Geometry: final body of the model. Coordinates: model frame, mm. Face numbers are marked on the shaded views. A direction names the side the tool comes from. Coordinates: 2 decimals unless noted, no trailing zeros. Loops run counter-clockwise (first coordinate to the right, second up) from the corner with the lowest first, then second, coordinate; pieces in that order, holes last. Notation, with made-up numbers: (28.25, 89) - (68.25, 89) arc R27 ccw to (68.25, 126) - close; hole circle Ø8 at (7, -12.75). An arc over 180 degrees is marked (long way). Answer in a Markdown table with one row per item.
from build123d import *

# Parameters (mm, degrees)
F1_DEPTH = 10.16
F3_DEPTH = 381
F5_DEPTH = 7.62


with BuildPart() as f1:
    # F0 (on Top) → F1 (new body)
    with BuildSketch(Plane.XY):
        with BuildLine():
            Line((-76.2, -76.2), (76.2, -76.2))
            ThreePointArc((76.2, -76.2), (94.1605122421, -68.7605122421), (101.6, -50.8))
            Line((101.6, -50.8), (101.6, 50.8))
            ThreePointArc((101.6, 50.8), (94.1605122421, 68.7605122421), (76.2, 76.2))
            Line((76.2, 76.2), (-76.2, 76.2))
            ThreePointArc((-76.2, 76.2), (-94.1605122421, 68.7605122421), (-101.6, 50.8))
            Line((-101.6, 50.8), (-101.6, -50.8))
            ThreePointArc((-101.6, -50.8), (-94.1605122421, -68.7605122421), (-76.2, -76.2))
        make_face()
    extrude(amount=-F1_DEPTH)

    # F2 (on face) → F3 (join)
    with BuildSketch(Plane.XY):
        with BuildLine():
            Line((-14.3209369853, 21.4582365006), (14.3209369853, 21.4582365006))
            Line((14.3209369853, 21.4582365006), (14.3209369853, 21.8244272492))
            ThreePointArc((14.3209369853, 21.8244272492), (6.4622604496, 29.6831037849), (14.3209369853, 37.5417803207))
            Line((14.3209369853, 37.5417803207), (14.3209369853, 37.9079710692))
            Line((14.3209369853, 37.9079710692), (-14.3209369853, 37.9079710692))
            Line((-14.3209369853, 37.9079710692), (-14.3209369853, 37.7833950656))
            ThreePointArc((-14.3209369853, 37.7833950656), (-8.5931660912, 35.410874679), (-6.2206457047, 29.6831037849))
            ThreePointArc((-6.2206457047, 29.6831037849), (-8.5931660912, 23.9553328908), (-14.3209369853, 21.5828125043))
            Line((-14.3209369853, 21.5828125043), (-14.3209369853, 21.4582365006))
        make_face()
        with BuildLine():
            ThreePointArc((14.3209369853, 37.5417803207), (6.4622604496, 29.6831037849), (14.3209369853, 21.8244272492))
            Line((14.3209369853, 21.8244272492), (14.3209369853, 37.5417803207))
        make_face()
        with BuildLine():
            Line((14.3209369853, 37.5417803207), (14.3209369853, 21.8244272492))
            ThreePointArc((14.3209369853, 21.8244272492), (19.8778604549, 24.1261803153), (22.1796135211, 29.6831037849))
            ThreePointArc((22.1796135211, 29.6831037849), (19.8778604549, 35.2400272545), (14.3209369853, 37.5417803207))
        make_face()
        with BuildLine():
            ThreePointArc((-14.3209369853, 37.7833950656), (-22.4212282659, 29.6831037849), (-14.3209369853, 21.5828125043))
            Line((-14.3209369853, 21.5828125043), (-14.3209369853, 37.7833950656))
        make_face()
        with BuildLine():
            Line((-14.3209369853, 37.7833950656), (-14.3209369853, 21.5828125043))
            ThreePointArc((-14.3209369853, 21.5828125043), (-8.5931660912, 23.9553328908), (-6.2206457047, 29.6831037849))
            ThreePointArc((-6.2206457047, 29.6831037849), (-8.5931660912, 35.410874679), (-14.3209369853, 37.7833950656))
        make_face()
    extrude(amount=F3_DEPTH)

    # F4 (on face) → F5 (join)
    with BuildSketch(Plane.XZ.offset(-21.4582365006)):
        with BuildLine():
            Line((-158.75, 254), (158.75, 254))
            ThreePointArc((158.75, 254), (160.5460512242, 254.7439487758), (161.29, 256.54))
            Line((161.29, 256.54), (161.29, 439.42))
            ThreePointArc((161.29, 439.42), (160.5460512242, 441.2160512242), (158.75, 441.96))
            Line((158.75, 441.96), (-158.75, 441.96))
            ThreePointArc((-158.75, 441.96), (-160.5460512242, 441.2160512242), (-161.29, 439.42))
            Line((-161.29, 439.42), (-161.29, 256.54))
            ThreePointArc((-161.29, 256.54), (-160.5460512242, 254.7439487758), (-158.75, 254))
        make_face()
    extrude(amount=F5_DEPTH)


solid = f1.part
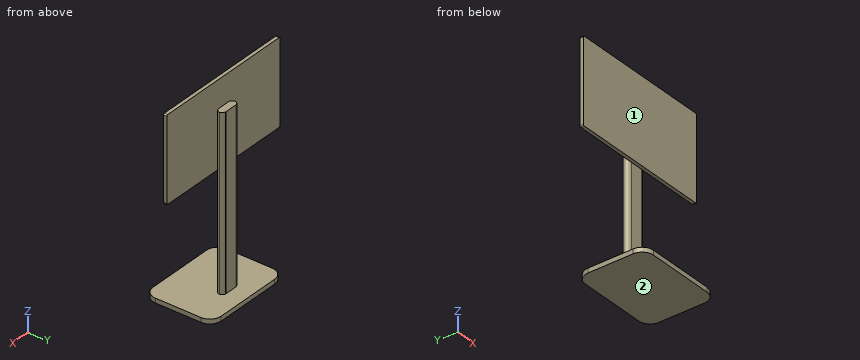
(1) Cut plane B-B on z = 227.5. Output: boundary loops of the cut face in (x, y), then the cut area to 3 significant figures.
Verdict:
| item | result |
|---|---|
| outline | (-14.32, 21.46) - (14.32, 21.46) - (14.32, 21.82) arc R7.86 ccw to (14.32, 37.54) - (14.32, 37.91) - (-14.32, 37.91) - (-14.32, 37.78) arc R8.1 ccw to (-14.32, 21.58) - close |
| area | 671 mm² |
(2) Access query for the marked faces 1 and 2. Directions: +Z, -Z, +X, -X, +Y, -Y. A direction counts if a zero-diameter tool reaches every point of the face in a straight line with its end or side. Return the directions, or none.
Verdict:
| item | result |
|---|---|
| face 1 | +Z, +X, -X, -Y |
| face 2 | -Z, +X, -X, +Y, -Y |
(3) Cut plane A-A on x = 57. Output: boundary loops of the cut face in (y, z).
Verdict:
| item | result |
|---|---|
| outline | (-76.2, -10.16) - (76.2, -10.16) - (76.2, 0) - (-76.2, 0) - close; (13.84, 254) - (21.46, 254) - (21.46, 441.96) - (13.84, 441.96) - close |
(4) Ray query, probe 1 along Z at (x, y) = (-9.5, 8.5); probe 2 along Y at (x, z) = (-2, 229); probe 3 along Y at (x, z) = (116, 410.5). Return the intervals inside material, ascending.
Verdict:
| item | result |
|---|---|
| probe 1 | z = -10.16 to 0 |
| probe 2 | y = 21.46 to 37.91 |
| probe 3 | y = 13.84 to 21.46 |
(5) Cut plane C-C on y = 4. Output: boundary loops of the cut face in (x, z).
Verdict:
| item | result |
|---|---|
| outline | (-101.6, -10.16) - (101.6, -10.16) - (101.6, 0) - (-101.6, 0) - close |
(6) Cut plane D-D on x = 113.5. Output: boundary loops of the cut face in (y, z), then the cut area to 3 significant figures.
Verdict:
| item | result |
|---|---|
| outline | (13.84, 254) - (21.46, 254) - (21.46, 441.96) - (13.84, 441.96) - close |
| area | 1,430 mm² |
(7) First-contact query: pin 1 Ø14.5 at (x, z) = (2, 165) entering from +Y; pin 2 Ø6 at (x, z) = (10, 70.5) entering from -Y; pin 3 Ø11 at (y, z) = (-14.5, -5) entering from -X. Flat tips, straight axial feed; report the tip coordinate or a pass-through.
Verdict:
| item | result |
|---|---|
| pin 1 | stops at y = 37.91 |
| pin 2 | stops at y = 21.46 |
| pin 3 | stops at x = -101.6 |
